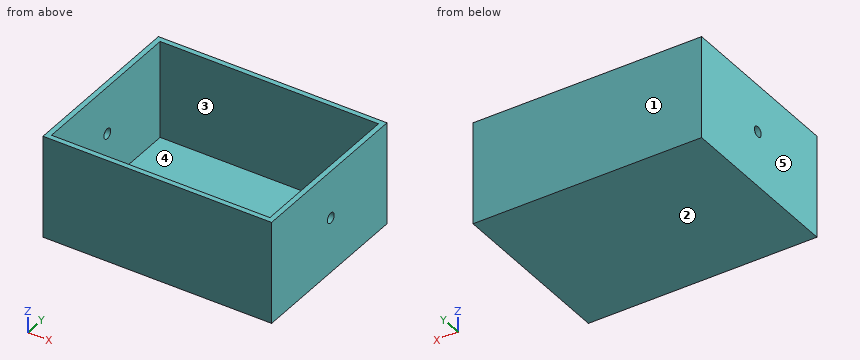
```python
from build123d import *

# Parameters (mm, degrees)
F0_W     = 111.455526
F0_H     = 85.127451
F1_DEPTH = 50
F2_T     = -2.5
F4_D     = 5


with BuildPart() as f1:
    # F0 (on Top) → F1 (new body)
    with BuildSketch(Plane.XY):
        with Locations((4.168613, -1.096998)):
            Rectangle(F0_W, F0_H)
    extrude(amount=F1_DEPTH)

    # F2
    f2_openings = [f1.faces().sort_by_distance(p)[0] for p in [
        (4.168613, -1.096997, 50),
    ]]
    offset(amount=F2_T, openings=f2_openings)

    # F4 (through all)
    with Locations(Plane.YZ.offset(59.896376)):
        with Locations((0, 26.930908)):
            Hole(F4_D / 2)


solid = f1.part
```
Work out the finished part from the listing and answer in its coordinate system (mm). Face numbers are marked on the shaded views. A direction names the side the tool comes from. Give positions to 0.01 mm unless a question says otherwise; leave off trailing zeros. Loops run counter-clockwise (first coordinate to the right, second up) from the corner with the lowest first, then second, coordinate; pieces in that order, holes last. Notation, with made-up numbers: M 74.25,72.25 L 133.25,72.25 A27 cw 133.25,96.25 Z; hole C -29,66.5 d6. An arc over 180 degrees is marked long. One line per item, written item: value. Start each with the question number.
1. Find section B-B (z = 20.5). Give the vertices of the cut face in (x, y), and give its area (3 significant figures).
2. Which of the six approach directions +Z, -Z, +X, -X, +Y, -Y give full straight-line access (tool end or side, diameter ignored) to the marked faces 4 and 5?
3. Determine the mould class of the marked faces 1, 2 and 3 for opening direction Y: released by +Y, released by -Y, zero draft, split by the parting line, or undercut.
4. Find section A-A (y = 0). Give the vertices of the cut face in (x, z).
5. Find section D-D (y = -18.5). Give the vertices of the cut face in (x, z).
6. Find section C-C (x = 31). Give the vertices of the cut face in (y, z).
7. Find the intervals of material crossed by probe 1 along Z at (x, y) = (59, 0); probe 2 along Y at (x, z) = (44, 41); probe 3 along X at (y, z) = (29.5, 26), in increasing order.
8. This flat-tipped pin is pushed along its axis until it touches: P1, Ø24, axis at x = 11.5, y = 11.5, coming from the +Z side. Where does it stop, or does it pass through?
Reported:
1. outline: M -51.56,-43.66 L 59.9,-43.66 L 59.9,41.47 L -51.56,41.47 Z; hole M -49.06,-41.16 L 57.4,-41.16 L 57.4,38.97 L -49.06,38.97 Z
1. area: 958 mm²
2. face 4: +Z
2. face 5: +Z, -Z, -X, +Y, -Y
3. face 1: released by +Y
3. face 2: zero draft
3. face 3: undercut
4. outline: M -51.56,0 L 59.9,0 L 59.9,24.43 L 57.4,24.43 L 57.4,2.5 L -49.06,2.5 L -49.06,24.43 L -51.56,24.43 Z; M -51.56,29.43 L -49.06,29.43 L -49.06,50 L -51.56,50 Z; M 57.4,29.43 L 59.9,29.43 L 59.9,50 L 57.4,50 Z
5. outline: M -51.56,0 L 59.9,0 L 59.9,50 L 57.4,50 L 57.4,2.5 L -49.06,2.5 L -49.06,50 L -51.56,50 Z
6. outline: M -43.66,0 L 41.47,0 L 41.47,50 L 38.97,50 L 38.97,2.5 L -41.16,2.5 L -41.16,50 L -43.66,50 Z
7. probe 1: z = 0 to 24.43, 29.43 to 50
7. probe 2: y = -43.66 to -41.16, 38.97 to 41.47
7. probe 3: x = -51.56 to -49.06, 57.4 to 59.9
8. P1: stops at z = 2.5
